The model under review builds one solid part; all positions refer to its coordinate system, in mm. A direction names the side the tool comes from. Give positions to 0.01 mm unless a question says otherwise; leave off trailing zeros. Write each loop counter-clockwise with the first axis right and the second up, starting at its lowest first coordinate (ties: lowest second). Pieces come first, ordered by that corner, then holes. Notation, with made-up numbers: (53.5, -21) - (59.5, -21) arc R14 cw to (59.5, -1) - close; hole circle Ø1 at (-6, 71.5). An arc over 180 degrees is marked (long way). Write item = value, one per line.
```python
from build123d import *

# Parameters (mm, degrees)
SKETCH_1_R               = 10.5
EXTRUDE_226_DEPTH        = 8
CUT_EXTRUDE_1_DEPTH      = 17.867127793
PATTERN_CIRCULAR_1_COUNT = 6
SKETCH_3_R               = 6
EXTRUDE_1_DEPTH          = 150
CHAMFER_1_SIZE           = 1


with BuildPart() as part:
    # Sketch 1 → Extrude 226 (new body)
    with BuildSketch(Plane.XY):
        Circle(SKETCH_1_R)
    extrude(amount=EXTRUDE_226_DEPTH)

    # Sketch 2 → Cut-Extrude 1 (cut, through all)
    with BuildSketch(Plane.XY.offset(8)):
        with BuildLine():
            Line((-9.5, 4.472135955), (-9.5, -4.472135955))
            ThreePointArc((-9.5, -4.472135955), (-10.5, 0), (-9.5, 4.472135955))
        make_face()
    cut_extrude_1 = extrude(amount=-CUT_EXTRUDE_1_DEPTH, mode=Mode.SUBTRACT)

    # Pattern Circular 1: Cut-Extrude 1 ×6 about axis
    pattern_circular_1_axis = Axis((0, 0, 0), (0, 0, 1))
    for i in range(1, PATTERN_CIRCULAR_1_COUNT):
        add(cut_extrude_1.rotate(pattern_circular_1_axis, i * 360 / PATTERN_CIRCULAR_1_COUNT), mode=Mode.SUBTRACT)

    # Sketch 3 → Extrude 1 (add)
    with BuildSketch(Plane.XY.offset(8)):
        Circle(SKETCH_3_R)
    extrude(amount=EXTRUDE_1_DEPTH)

    # Chamfer 1
    chamfer_1_edges = [part.edges().sort_by_distance(p)[0] for p in [
        (-6, 0, 158),
    ]]
    chamfer(chamfer_1_edges, length=CHAMFER_1_SIZE)


solid = part.part
```
1. For line 1 (Z direction, x = 8, y = 4.5); line 2 (X direction, y = 4, z = 144); line 3 (X direction, y = -3.25, z = 88.5), list the stretches that pass through material, from the lowest coordinate up. Write a range as from..to.
Findings below:
line_1 = 0..8
line_2 = -4.47..4.47
line_3 = -5.04..5.04
2. Insertion check: P1, Ø1.5, axis at x = -2.5, z = 140.5, coming from the -Y side; P2, Ø2, axis at x = 5.5, y = -4, coming from the -Z side; P3, Ø5, axis at y = -2, z = 127, coming from the +X side; P4, Ø4, axis at y = -5.5, z = 95, coming from the -X side. Each pin has a flat end and moves straight along its axis. Give the tip position at first contact, or say it passes through.
Findings below:
P1 = -5.74
P2 = 0
P3 = 6
P4 = -4.87
3. Take a section at A-A on y = 0. Give the boundary of the cut face in (x, z).
Findings below:
outline = (-9.5, 0) - (9.5, 0) - (9.5, 8) - (6, 8) - (6, 157) - (5, 158) - (-5, 158) - (-6, 157) - (-6, 8) - (-9.5, 8) - close
4. Machinability: for faces 1 (the flat face through (-4, -5, 8)), 2 (the flat face through (-4.696, 8.259, 4.056)), which of the approach directions +Z, -Z, +X, -X, +Y, -Y give a long, thin tool a straight path to every point of the face, cutting with its end or side? Answer none if there is none.
Findings below:
face_1 = +Z
face_2 = +Z, -Z, -X, +Y
5. Take a section at B-B on z = 118. Give the boundary of the cut face in (x, y), and give its area (3 significant figures).
Findings below:
outline = circle Ø12 at (0, 0)
area = 113 mm²
